Input: part model. Units: mm. Frame: model coordinates. Face numbers are marked on the shaded views. A direction names the side the tool comes from. Round coordinates to 2 decimals unless told otherwise and drop trailing zeros. Order: outer loops, then holes, each group sorted by start corner. A loop starts at its lowest first (then second) coordinate and runs counter-clockwise, first axis right, second up. Notation, with made-up numbers: M 73.5,36 L 98.5,36 A12 ccw 98.5,44 Z; hole C 59.5,14.25 d11. An arc over 180 degrees is marked long. One line per question, with ' | ' between items.
```python
from build123d import *

# Parameters (mm, degrees)
SKETCH_1_R           = 0.65
EXTRUDE_1_DEPTH      = 10
EXTRUDE_1_DEPTH_BACK = 8
SKETCH_2_R           = 2.6
EXTRUDE_3_DEPTH      = 4.5
EXTRUDE_3_DEPTH_BACK = 4.5


with BuildPart() as part:
    # Эскиз1 → Бобышка-Вытянуть1 (new body, two sides)
    with BuildSketch(Plane.XY) as extrude_1_sk:
        Circle(SKETCH_1_R)
    extrude(amount=EXTRUDE_1_DEPTH)
    extrude(extrude_1_sk.sketch, amount=-EXTRUDE_1_DEPTH_BACK)

    # Эскиз2 → Бобышка-Вытянуть3 (add, two sides)
    with BuildSketch(Plane.XY) as extrude_3_sk:
        Circle(SKETCH_2_R)
    extrude(amount=EXTRUDE_3_DEPTH)
    extrude(extrude_3_sk.sketch, amount=-EXTRUDE_3_DEPTH_BACK)


solid = part.part
```
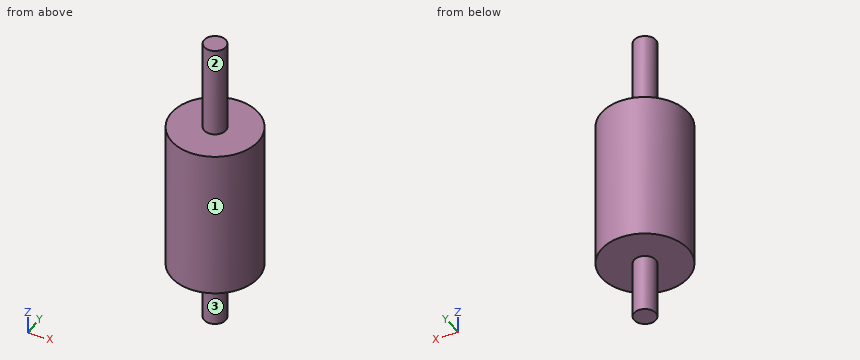
Item 1: Access query for the marked faces 1, 2 and 3. Directions: +Z, -Z, +X, -X, +Y, -Y. A direction counts if a zero-diameter tool reaches every point of the face in a straight line with its end or side. Return the directions, or none.
Report:
face 1: +Z, -Z | face 2: +Z | face 3: -Z
Item 2: Section query C-C, the plane z = 6.5. Return loops of the section in (x, y).
Report:
outline: C 0,0 d1.3
Item 3: Section query D-D, the plane y = 1. Return loops of the section in (x, z), plus the area to 3 significant figures.
Report:
outline: M -2.4,-4.5 L 2.4,-4.5 L 2.4,4.5 L -2.4,4.5 Z | area: 43.2 mm²
Item 4: Line query: line 1 along Z through (x, y) = (-2.05, -0.4); line 2 along Y through (x, z) = (2.25, 0.25); line 3 along X through (y, z) = (-1.65, 4.25). Output: solid intervals per line, ascending. Write a range as from..to.
Report:
line 1: -4.5..4.5 | line 2: -1.3..1.3 | line 3: -2.01..2.01
Item 5: First-contact query: pin 1 (3 mm diameter, centred on y = 0.5, z = -1, fed in from +X); pin 2 (1 mm diameter, centred on x = 2, z = -6, fed in from +Y); pin 3 (1.5 mm diameter, centred on x = -2, z = 2.5, fed in from +Y); pin 4 (1 mm diameter, centred on x = -1, z = -1.5, fed in from +Y). Flat tips, straight axial feed; report the tip coordinate or a pass-through.
Report:
pin 1: x = 2.6 | pin 2: through | pin 3: y = 2.28 | pin 4: y = 2.55
Item 6: Section query A-A, the plane y = 0. Return loops of the section in (x, z).
Report:
outline: M -2.6,-4.5 L -0.65,-4.5 L -0.65,-8 L 0.65,-8 L 0.65,-4.5 L 2.6,-4.5 L 2.6,4.5 L 0.65,4.5 L 0.65,10 L -0.65,10 L -0.65,4.5 L -2.6,4.5 Z
